Print and shaded views of the part. All mm, measured from the part's lowest x, y and z. Give positions to 0.01 mm unless a question says otherwise; leave off trailing zeros. Loops run counter-clockwise (first coordinate to the right, second up) from the corner with the lowest first, then second, coordinate; pieces in that order, holes last. Notation, with made-up numbers: M -34,61 L -8,61 A19 ccw -8,76 Z; hole C 24.5,85 d2. An arc over 180 degrees is marked long. Put each result on its own line as item: value. Start each with the question number.
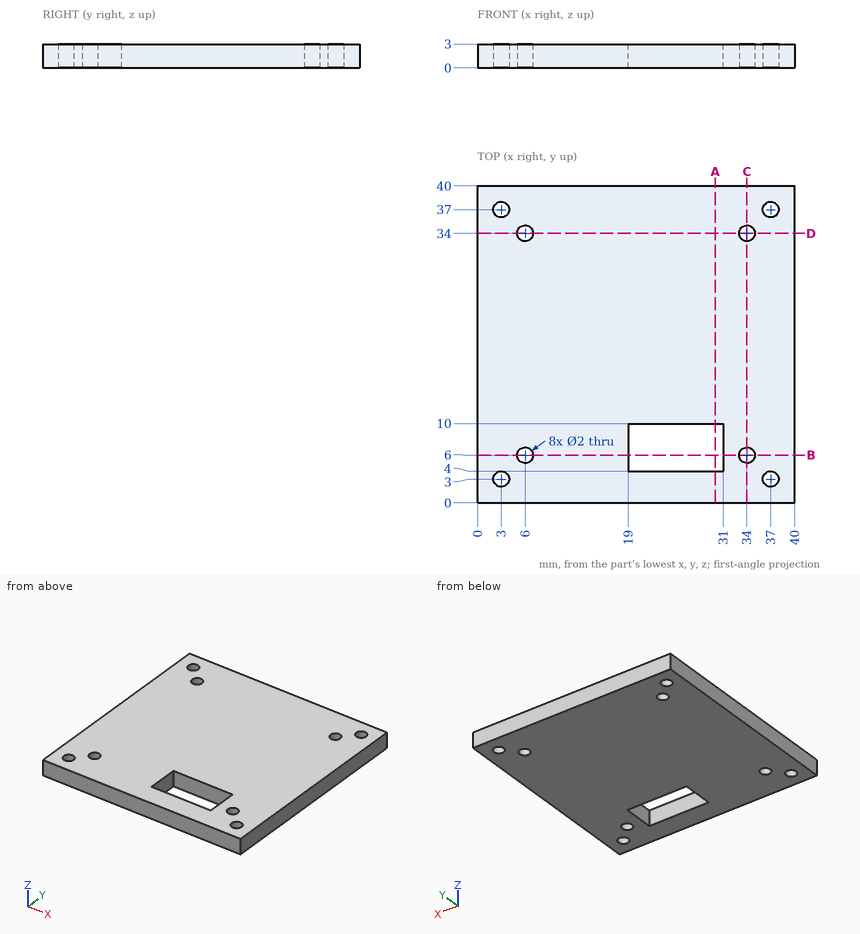
1) Band-saw the part on A-A on x = 30. Give the cut face in (y, z).
2) Band-saw the part on B-B on y = 6. Give the cut face in (x, z), then the cut area to 3 significant figures.
3) Band-saw the part on C-C on x = 34. Give the cut face in (y, z), then the cut area to 3 significant figures.
4) Wall check: L1, parallel to Y at x = 34, z = 1.35; L2, parallel to Y at x = 3, z = 0.7; L3, parallel to Y at x = 28, z = 2.4. Give the ranges that are in metal, low to high.
Evaluation:
1. outline: M 0,0 L 4,0 L 4,3 L 0,3 Z; M 10,0 L 40,0 L 40,3 L 10,3 Z
2. outline: M 0,0 L 5,0 L 5,3 L 0,3 Z; M 7,0 L 19,0 L 19,3 L 7,3 Z; M 31,0 L 33,0 L 33,3 L 31,3 Z; M 35,0 L 40,0 L 40,3 L 35,3 Z
2. area: 72.0 mm2
3. outline: M 0,0 L 5,0 L 5,3 L 0,3 Z; M 7,0 L 33,0 L 33,3 L 7,3 Z; M 35,0 L 40,0 L 40,3 L 35,3 Z
3. area: 108 mm2
4. L1: 0 to 5, 7 to 33, 35 to 40
4. L2: 0 to 2, 4 to 36, 38 to 40
4. L3: 0 to 4, 10 to 40
